from build123d import *

# Parameters (mm, degrees)
F0_W      = 32
F0_H      = 42
F1_DEPTH  = 46
F2_W      = 33
F2_H      = 29.25
F3_DEPTH  = 42.001
F4_SIZE   = 26
F5_R      = 1
F6_DEPTH  = 25
F7_W      = 46
F7_H      = 7
F7_H_2    = 3.5
F8_DEPTH  = 10
F9_SIZE   = 5
F10_R     = 1
F11_R     = 0.75
F12_DEPTH = 5


with BuildPart() as f1:
    # F0 (on Right) → F1 (new body)
    with BuildSketch(Plane.YZ):
        with Locations((16, 21)):
            Rectangle(F0_W, F0_H)
    extrude(amount=-F1_DEPTH)

    # F2 (on Top) → F3 (cut, through all)
    with BuildSketch(Plane.XY):
        with Locations((-23, 14.625)):
            Rectangle(F2_W, F2_H)
    extrude(amount=F3_DEPTH, mode=Mode.SUBTRACT)

    # F4
    f4_edges = [f1.edges().sort_by_distance(p)[0] for p in [
        (-42.75, 0, 42),
        (-3.25, 0, 42),
    ]]
    chamfer(f4_edges, length=F4_SIZE)

    # F5 (on face) → F6 (cut)
    with BuildSketch(Plane.XZ.offset(-29.25)):
        with Locations((-35.0738482888, 33.0738482888)):
            Circle(F5_R)
        with Locations((-10.9261517112, 33.0738482888)):
            Circle(F5_R)
        with Locations((-35.0738482888, 8.9261517112)):
            Circle(F5_R)
        with Locations((-10.9261517112, 8.9261517112)):
            Circle(F5_R)
    extrude(amount=-F6_DEPTH, mode=Mode.SUBTRACT)

    # F7 (on face) → F8 (join)
    with BuildSketch(Plane(origin=(0, 32, 0), x_dir=(-1, 0, 0), z_dir=(0, 1, 0))):
        with Locations((23, 41.5)):
            Rectangle(F7_W, F7_H)
        with Locations((23, 1.75)):
            Rectangle(F7_W, F7_H_2)
    extrude(amount=-F8_DEPTH)

    # F9
    f9_edges = [f1.edges().sort_by_distance(p)[0] for p in [
        (-42.75, 22, 38),
        (-3.25, 22, 38),
    ]]
    chamfer(f9_edges, length=F9_SIZE)

    # F10
    f10_edges = [f1.edges().sort_by_distance(p)[0] for p in [
        (-39.5, 29.25, 20.75),
        (-6.5, 29.25, 20.75),
        (-23, 29.25, 38),
        (-23, 29.25, 3.5),
        (-39.5, 25.625, 3.5),
        (-6.5, 25.625, 3.5),
    ]]
    fillet(f10_edges, radius=F10_R)

    # F11 (on face) → F12 (cut)
    with BuildSketch(Plane(origin=(0, 0, 0), x_dir=(1, 0, 0), z_dir=(0, 0, -1))):
        with Locations((-42.75, -4)):
            Circle(F11_R)
        with Locations((-42.75, -28.5)):
            Circle(F11_R)
        with Locations((-3.25, -28.5)):
            Circle(F11_R)
        with Locations((-3.25, -4)):
            Circle(F11_R)
    extrude(amount=-F12_DEPTH, mode=Mode.SUBTRACT)


solid = f1.part
Input: part model. Units: mm. Frame: model coordinates. A direction names the side the tool comes from. Coordinates: 2 decimals unless noted, no trailing zeros. Order: outer loops, then holes, each group sorted by start corner. A loop starts at its lowest first (then second) coordinate and runs counter-clockwise, first axis right, second up. Notation, with made-up numbers: M 53.5,8.25 L 111.5,8.25 A12 ccw 111.5,19.25 Z; hole C 21.5,51.5 d3. An arc over 180 degrees is marked long. Answer in a Markdown table with one row per item.
(1) Material intervals for line 1 (X direction, y = 9.5, z = 14); line 2 (Y direction, x = -3.25, z = 1.2); line 3 (X direction, y = 4, z = 3), sorted ascending. Write a range as [from, to].
Numbers:
| item | result |
|---|---|
| line 1 | x = [-46, -39.5], [-6.5, 0] |
| line 2 | y = [0, 3.25], [4.75, 27.75], [29.25, 32] |
| line 3 | x = [-46, -43.5], [-42, -39.5], [-6.5, -4], [-2.5, 0] |
(2) Contact query for flat-ended pins moving along their axis: pin 1 Ø0.9 at (x, y) = (-42.75, 28.5) entering from -Z; pin 2 Ø6 at (x, z) = (-10.5, 5) entering from -Y; pin 3 Ø2.5 at (x, y) = (-42.75, 4) entering from +Z. Output: stop coordinate, or through.
Numbers:
| item | result |
|---|---|
| pin 1 | stops at z = 5 |
| pin 2 | stops at y = 22 |
| pin 3 | stops at z = 21.25 |
(3) Section query A-A, the plane y = 5.5. Output: boundary loops of the cut face in (x, z), plus the area to 4 significant figures.
Numbers:
| item | result |
|---|---|
| outline | M -46,0 L -39.5,0 L -39.5,21.5 L -46,21.5 Z; M -6.5,0 L 0,0 L 0,21.5 L -6.5,21.5 Z |
| area | 279.5 mm^2 |
(4) Draft query along Y for faces 1 (the flat face through (-23, 32, 22)), 2 (the flat face through (-23, 25, 3.5)), 3 (the flat face through (-3, 9, 25)), 4 (the flat face through (-43, 28, 5)). Return one class per face: pulls with the +Y half, pulls with the -Y half, needs draft (parallel to the pull), parting line crosses it, or undercut.
Numbers:
| item | result |
|---|---|
| face 1 | pulls with the +Y half |
| face 2 | needs draft |
| face 3 | pulls with the -Y half |
| face 4 | undercut |
(5) Section query C-C, the plane x = -42.75. Output: boundary loops of the cut face in (y, z), plus the area to 3 significant figures.
Numbers:
| item | result |
|---|---|
| outline | M 0,0 L 3.25,0 L 3.25,5 L 4.75,5 L 4.75,0 L 27.75,0 L 27.75,5 L 29.25,5 L 29.25,0 L 32,0 L 32,45 L 22,45 L 22,43 L 18.46,34.46 L 0,16 Z |
| area | 1,040 mm^2 |
(6) Access query for faces 5 (the flat face through (-23, 22, 2)), 6 (the flat face through (-3, 28, 5)), 7 (the flat face through (-23, 29.25, 21)). Directions: +Z, -Z, +X, -X, +Y, -Y. A direction counts if a zero-diameter tool reaches every point of the face in a straight line with its end or side. Return the directions, or none.
Numbers:
| item | result |
|---|---|
| face 5 | +Z, -Z, -Y |
| face 6 | -Z |
| face 7 | -Y |
(7) Section query B-B, the plane z = 31. Output: boundary loops of the cut face in (x, y).
Numbers:
| item | result |
|---|---|
| outline | M -46,15 L -39.5,15 L -39.5,28.25 A1 cw -38.5,29.25 L -7.5,29.25 A1 cw -6.5,28.25 L -6.5,15 L 0,15 L 0,32 L -46,32 Z |
(8) Section query D-D, the plane y = 23.5. Output: boundary loops of the cut face in (x, z).
Numbers:
| item | result |
|---|---|
| outline | M -46,0 L 0,0 L 0,45 L -46,45 Z; hole M -39.5,4.5 A1 ccw -38.5,3.5 L -7.5,3.5 A1 ccw -6.5,4.5 L -6.5,38 L -39.5,38 Z |
